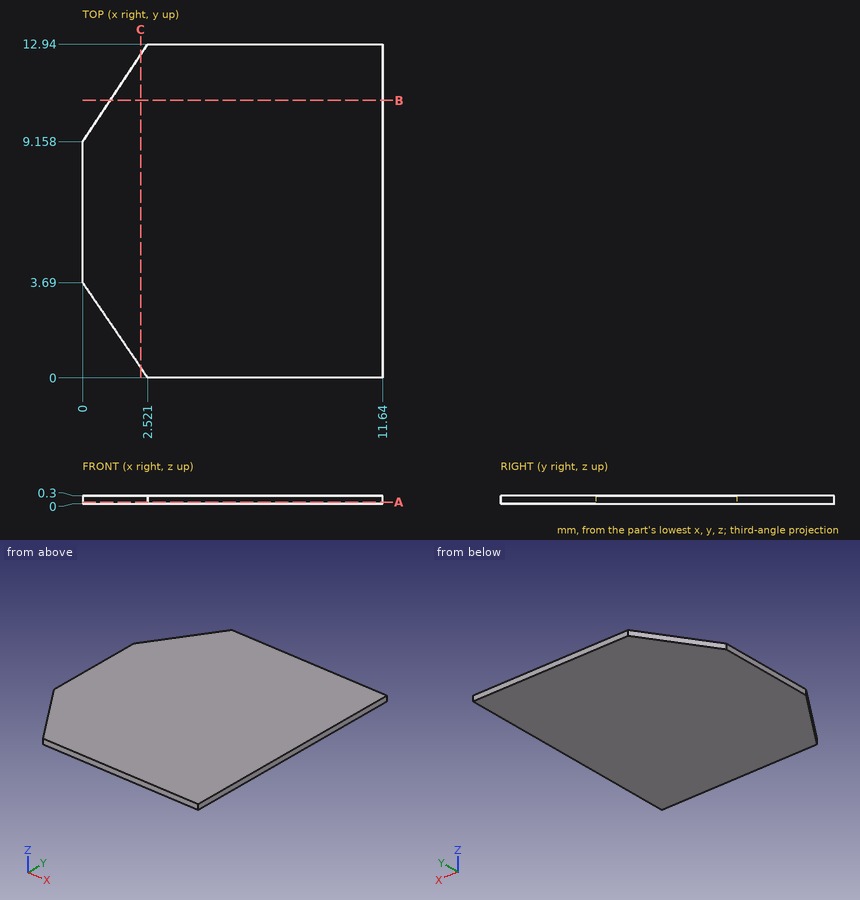
Study the drawing (mm; zero at the part's minimum x, y, z) and answer. Coordinates: 2 decimals unless noted, no trailing zeros. Loops run counter-clockwise (first coordinate to the right, second up) from the corner with the lowest first, then second, coordinate; pieces in that order, holes last. Notation, with made-up numbers: M 57,10.5 L 83,10.5 A25 cw 83,37.5 Z; hole C 49.25,-10 d4. An arc over 180 degrees is marked long. Answer in a Markdown table with one row per item. Add a question column.
1. Find section C-C, the plane x = 2.25. Write down the section's boundary in (y, z), then the cut area to 3 significant figures.
2. Find section A-A, the plane z = 0.05. Write down the section's boundary in (x, y).
3. Find section B-B, the plane y = 10.75. Write down the section's boundary in (x, z).
4. Consider L1, parallel to X at y = 2.75, z = 0.1; L2, parallel to Y at x = 0.5, z = 0.05; L3, parallel to X at y = 2.5, z = 0.1. Determine where each line is inside the solid, lowest interval first.
Reported:
| question | item | result |
|---|---|---|
| 1 | outline | M 0.4,0 L 12.53,0 L 12.53,0.3 L 0.4,0.3 Z |
| 1 | area | 3.64 mm^2 |
| 2 | outline | M 0,3.69 L 2.52,0 L 11.64,0 L 11.64,12.94 L 2.52,12.94 L 0,9.16 Z |
| 3 | outline | M 1.06,0 L 11.64,0 L 11.64,0.3 L 1.06,0.3 Z |
| 4 | L1 | x = 0.64 to 11.64 |
| 4 | L2 | y = 2.96 to 9.91 |
| 4 | L3 | x = 0.81 to 11.64 |
